CAD build for the part. Positions are in the model's coordinates, mm. A direction names the side the tool comes from. Round coordinates to 2 decimals unless told otherwise and drop trailing zeros. Write each loop counter-clockwise with the first axis right and the second up, starting at its lowest first coordinate (ties: lowest second). Pieces come first, ordered by that corner, then holes. Notation, with made-up numbers: (40.5, -9) - (83.5, -9) arc R24 ccw to (83.5, 11) - close; hole circle Ø10 at (73.5, 43.5). An arc over 180 degrees is marked (long way). Put each result on its own line as item: value. Start each with the question number.
Item 1: Cut at B-B (z = 1.5). Give the cut face in (x, y).
Item 2: Cut at C-C (x = -6.5). Give the cut face in (y, z).
Item 3: Cut at D-D (y = 3.75). Give the cut face in (x, z), and give its area (3 significant figures).
Item 4: Pin check, flat tips, straight feed: pin 1 Ø4.5 at (x, z) = (-6.5, 0) entering from -Y; pin 2 Ø1 at (y, z) = (-5.5, -2) entering from +X. Stop position of each tip, or through.
Item 5: Drill centre lines: line 1 (Z direction, x = 1.25, y = -0.25); line 2 (X direction, y = 6.25, z = 1.5); line 3 (Z direction, x = -5.5, y = 6). Where is each one in solid material? Low to high. Write a range as from..to.
Item 6: Mould opens along X. For faces 3 (the cylindrical face through (4.963, 0.088, -5.726)), 4 (the flat face through (0, 0, 0)), 5 (the flat face through (0, 0, 7.5)) say: released by +X, released by -X, zero draft, split by the parting line, or undercut.
Item 7: 3-axis set-ups, long thin cutter, end or side, ignore diameter. For faces 1 (the flat face through (-12.5, 0, 0)), 2 (the flat face through (4.8, 0.1, 4)): which of +Z, -Z, +X, -X, +Y, -Y reach the whole face in a straight line?
Item 8: Cut at A-A (y = 0). Give the cut face in (x, z).
```python
from build123d import *

# Parameters (mm, degrees)
CROQUIS1_W              = 15
CROQUIS1_H              = 15
SALIENTE_EXTRUIR1_DEPTH = 12.5
CROQUIS2_R              = 2.5
CROQUIS2_W              = 25
CROQUIS2_H              = 8
CORTAR_EXTRUIR1_DEPTH   = 21.916500663
CROQUIS3_R              = 2
CORTAR_EXTRUIR2_DEPTH   = 21.916500663


with BuildPart() as part:
    # Croquis1 → Saliente-Extruir1 (new, symmetric)
    with BuildSketch(Plane(origin=(0, 0, 0), x_dir=(0, 0, -1), z_dir=(1, 0, 0))):
        Rectangle(CROQUIS1_W, CROQUIS1_H)
    extrude(amount=SALIENTE_EXTRUIR1_DEPTH, both=True)

    # Croquis2 → Cortar-Extruir1 (cut, through all)
    with BuildSketch(Plane(origin=(0, 7.5, 0), x_dir=(1, 0, 0), z_dir=(0, 1, 0))):
        with Locations(Location((-6.5, 0, 0), (0, 0, 270))):
            Circle(CROQUIS2_R)
        with Locations((12.5, 0)):
            Rectangle(CROQUIS2_W, CROQUIS2_H)
    extrude(amount=-CORTAR_EXTRUIR1_DEPTH, mode=Mode.SUBTRACT)

    # Croquis3 → Cortar-Extruir2 (cut, through all)
    with BuildSketch(Plane.XY.offset(7.5)):
        with Locations((6.961549082, 0)):
            Circle(CROQUIS3_R)
    extrude(amount=-CORTAR_EXTRUIR2_DEPTH, mode=Mode.SUBTRACT)


solid = part.part
```
Output values:
1. outline: (-12.5, -7.5) - (-8.5, -7.5) - (-8.5, 7.5) - (-12.5, 7.5) - close; (-4.5, -7.5) - (0, -7.5) - (0, 7.5) - (-4.5, 7.5) - close
2. outline: (-7.5, -7.5) - (7.5, -7.5) - (7.5, -2.5) - (-7.5, -2.5) - close; (-7.5, 2.5) - (7.5, 2.5) - (7.5, 7.5) - (-7.5, 7.5) - close
3. outline: (-12.5, -7.5) - (12.5, -7.5) - (12.5, -4) - (0, -4) - (0, 4) - (12.5, 4) - (12.5, 7.5) - (-12.5, 7.5) - close; hole circle Ø5 at (-6.5, 0)
3. area: 255 mm2
4. pin 1: through
4. pin 2: x = 0
5. line 1: -7.5..-4, 4..7.5
5. line 2: -12.5..-8.5, -4.5..0
5. line 3: -7.5..-2.29, 2.29..7.5
6. face 3: undercut
6. face 4: released by +X
6. face 5: zero draft
7. face 1: +Z, -Z, -X, +Y, -Y
7. face 2: +X, +Y, -Y
8. outline: (-12.5, -7.5) - (4.96, -7.5) - (4.96, -4) - (0, -4) - (0, 4) - (4.96, 4) - (4.96, 7.5) - (-12.5, 7.5) - close; (8.96, -7.5) - (12.5, -7.5) - (12.5, -4) - (8.96, -4) - close; (8.96, 4) - (12.5, 4) - (12.5, 7.5) - (8.96, 7.5) - close; hole circle Ø5 at (-6.5, 0)
